Source: three-view drawing plus pictorial views. Frame: mm from the lowest corner of the part. A direction names the side the tool comes from. Give positions to 0.01 mm unless a question says otherwise; leave off trailing zeros. Order: outer loops, then holes, each group sorted by start corner. A loop starts at its lowest first (then second) coordinate and runs counter-clockwise, first axis right, second up. Notation, with made-up numbers: (77.5, 59) -> (111.5, 59) arc R17 ccw to (111.5, 77) -> close; hole circle Ø11 at (59, 28.25). An arc over 180 degrees is marked (long way). One line per question, with ' | ' between items.
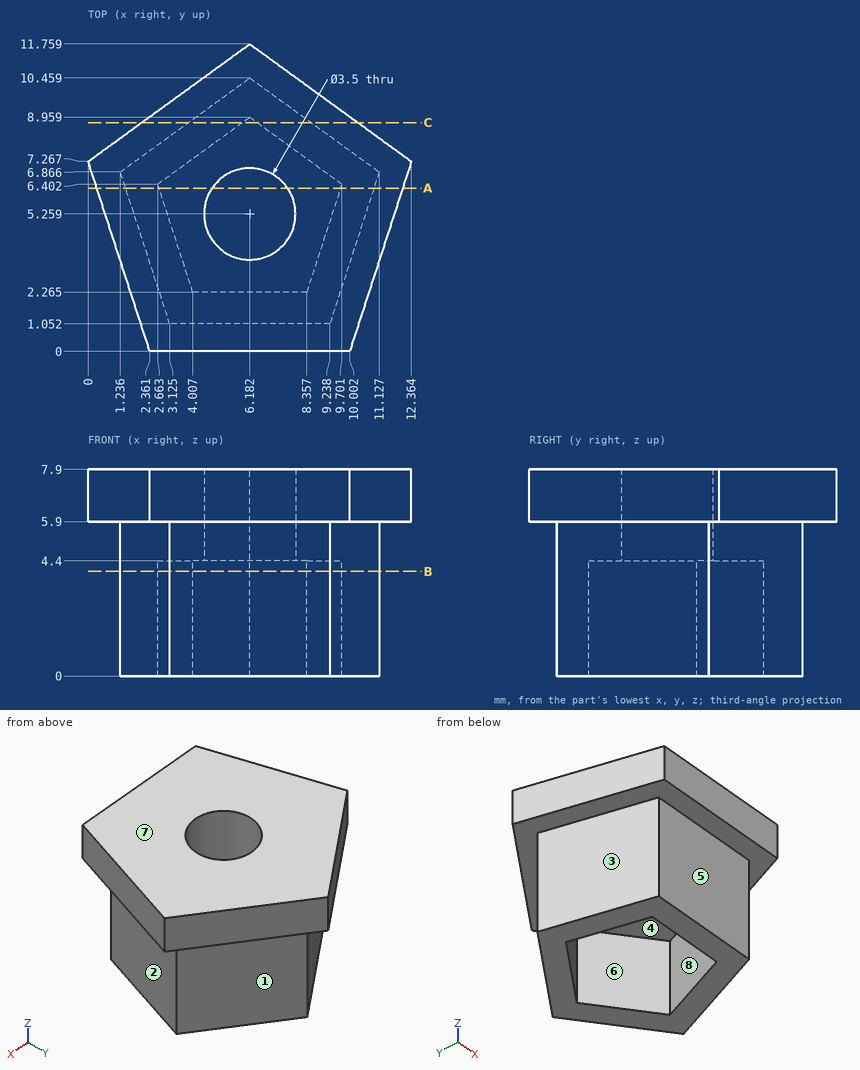
1) Section A-A on y = 6.25. Return loops of the section in (x, z) (1 decimal).
Check result:
outline: (0.3, 5.9) -> (1.4, 5.9) -> (1.4, 0) -> (2.7, 0) -> (2.7, 4.4) -> (4.7, 4.4) -> (4.7, 7.9) -> (0.3, 7.9) -> close; (7.6, 4.4) -> (9.7, 4.4) -> (9.7, 0) -> (10.9, 0) -> (10.9, 5.9) -> (12, 5.9) -> (12, 7.9) -> (7.6, 7.9) -> close
2) Contact query for flat-ended pins moving along their axis: pin 1 Ø1.5 at (y, z) = (6, 2) entering from +X; pin 2 Ø3 at (x, z) = (7, 2) entering from -Y; pin 3 Ø3.5 at (x, y) = (6, 6.5) entering from -Z. Output: stop coordinate, or through.
Check result:
pin 1: stops at x = 11.09 | pin 2: stops at y = 1.05 | pin 3: stops at z = 4.4
3) Section C-C on y = 8.75. Return loops of the section in (x, z) (1 decimal).
Check result:
outline: (2, 5.9) -> (3.8, 5.9) -> (3.8, 0) -> (5.9, 0) -> (5.9, 4.4) -> (6.5, 4.4) -> (6.5, 0) -> (8.5, 0) -> (8.5, 5.9) -> (10.3, 5.9) -> (10.3, 7.9) -> (2, 7.9) -> close
4) Set-up query: the marked faces 1, 2, 3 and 4. Return all of +Z, -Z, +X, -X, +Y, -Y with unobstructed straight access to the full face (end or side cutting, diameter ignored); none if empty.
Check result:
face 1: -Z, +X, +Y | face 2: -Z, +X, -Y | face 3: -Z, -X, -Y | face 4: -Z
5) Pull-direction query (Y, two-part tool) for the marked faces 5, 6, 7 and 8; classes: +Y half, -Y half, draft (parallel to the pull), parting line (faces both ways), or undercut.
Check result:
face 5: -Y half | face 6: undercut | face 7: draft | face 8: undercut
6) Section B-B on z = 4. Return loops of the section in (x, y) (1 decimal).
Check result:
outline: (1.2, 6.9) -> (3.1, 1.1) -> (9.2, 1.1) -> (11.1, 6.9) -> (6.2, 10.5) -> close; hole (2.7, 6.4) -> (4, 2.3) -> (8.4, 2.3) -> (9.7, 6.4) -> (6.2, 9) -> close
7) Material intervals for probe 1 along Z at (x, y) = (3.5, 6.75); probe 2 along Z at (x, y) = (8.25, 9.5); probe 3 along X at (y, z) = (8.25, 1.25) (1 decimal), sorted ascending. Write a range as from..to.
Check result:
probe 1: z = 4.4..7.9 | probe 2: z = 5.9..7.9 | probe 3: x = 3.1..5.2, 7.2..9.2
